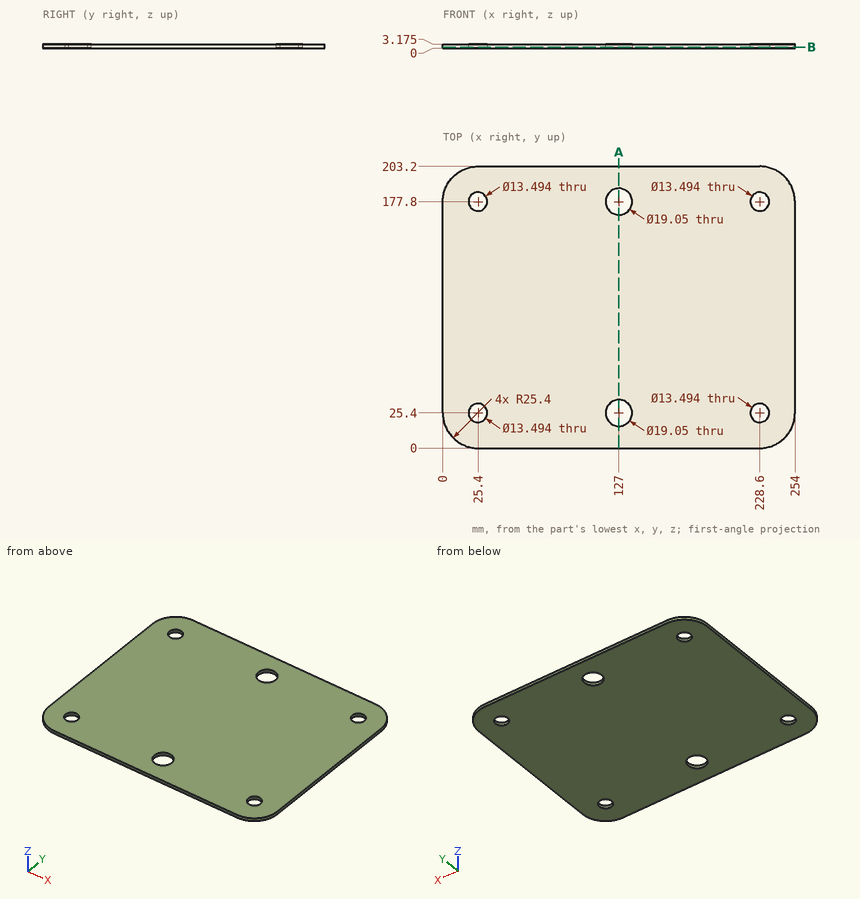
Part print with two shaded views. Sizes in mm from the minimum x, y, z corner. Round coordinates to 2 decimals unless told otherwise and drop trailing zeros. Order: outer loops, then holes, each group sorted by start corner. A loop starts at its lowest first (then second) coordinate and runs counter-clockwise, first axis right, second up. Notation, with made-up numbers: (-23, 64.25) -> (-18, 64.25) arc R16 ccw to (-18, 84.25) -> close; hole circle Ø7 at (25, 55.5). An arc over 180 degrees is marked (long way). Use one line per item in the form item = value.
Item 1: Cut at B-B, the plane z = 0.9. Give the number of separate pieces and of enclosed holes in the cut face, and give its area (3 significant figures).
Returned:
separate_pieces = 1
enclosed_holes = 6
area = 49,900 mm^2
Item 2: Drill centre lines: line 1 (X direction, y = 25, z = 1.5) (1 decimal); line 2 (Y direction, x = 126, z = 2.3); line 3 (Y direction, x = 25.4, z = 2.2). Where is each one in solid material? Low to high.
Returned:
line_1 = 0 to 18.7, 32.1 to 117.5, 136.5 to 221.9, 235.3 to 254
line_2 = 0 to 15.93, 34.87 to 168.33, 187.27 to 203.2
line_3 = 0 to 18.65, 32.15 to 171.05, 184.55 to 203.2
Item 3: Cut at A-A, the plane x = 127. Write the cut outline in (y, z) (1 decimal).
Returned:
outline = (0, 0) -> (15.9, 0) -> (15.9, 3.2) -> (0, 3.2) -> close; (34.9, 0) -> (168.3, 0) -> (168.3, 3.2) -> (34.9, 3.2) -> close; (187.3, 0) -> (203.2, 0) -> (203.2, 3.2) -> (187.3, 3.2) -> close
Item 4: Flat gauge pin, fed straight in: pin 1 Ø1.5 at (y, z) = (102.5, 2.5) entering from -X. Where does the tip first touch, or does it go through?
Returned:
pin_1 = 0
